```python
from build123d import *

# Parameters (mm, degrees)
SKETCH1_W           = 37
SKETCH1_H           = 20
BOSS_EXTRUDE1_DEPTH = 8
FILLET1_R           = 2
FILLET2_R           = 2


with BuildPart() as part:
    # Sketch1 → Boss-Extrude1 (new body)
    with BuildSketch(Plane(origin=(0, 0, 0), x_dir=(1, 0, 0), z_dir=(0, 1, 0))):
        with Locations((18.5, 10)):
            Rectangle(SKETCH1_W, SKETCH1_H)
    extrude(amount=BOSS_EXTRUDE1_DEPTH)

    # Fillet1
    fillet1_edges = [part.edges().sort_by_distance(p)[0] for p in [
        (18.5, 8, 0),
    ]]
    fillet(fillet1_edges, radius=FILLET1_R)

    # Fillet2
    fillet2_edges = [part.edges().sort_by_distance(p)[0] for p in [
        (18.5, 8, -20),
        (18.5, 0, -20),
        (18.5, 0, 0),
        (0, 4, -20),
        (37, 4, -20),
    ]]
    fillet(fillet2_edges, radius=FILLET2_R)


solid = part.part
```
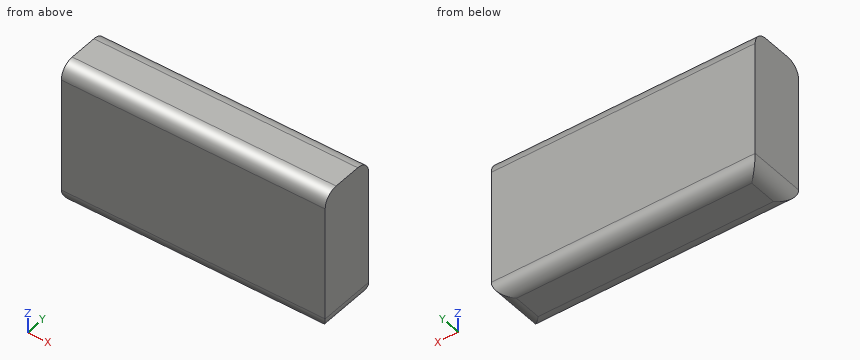
Read the model definition and answer for the solid it produces. Units are mm, in the model's axes. Coordinates: 2 decimals unless noted, no trailing zeros. Loops run counter-clockwise (first coordinate to the right, second up) from the corner with the lowest first, then second, coordinate; pieces in that order, holes last.
(1) The part is cut by section A-A (x = 27). Determine the outline of the cut face in (y, z).
Solution:
outline: (0, -18) arc R2 ccw to (2, -20) - (6, -20) arc R2 ccw to (8, -18) - (8, -2) arc R2 ccw to (6, 0) - (2, 0) arc R2 ccw to (0, -2) - close
(2) The part is cut by section B-B (y = 1). Determine the outline of the cut face in (x, z), and give its area (3 significant figures).
Solution:
outline: (0, -18) arc R2 ccw to (1, -19.73) - (36, -19.73) arc R2 ccw to (37, -18) - (37, -0.27) - (0, -0.27) - close
area: 719 mm2
(3) Consider line 1 along Z through (x, y) = (7, 0.5); line 2 along Z through (x, y) = (32, 1). Determine where each line is inside the solid, lowest interval first.
Solution:
line 1: z = -19.32 to -0.68
line 2: z = -19.73 to -0.27
